from build123d import *

# Parameters (mm, degrees)
F1_DEPTH = 254
F2_T     = -2.54
F4_DEPTH = 25.4


with BuildPart() as f1:
    # F0 (on Right) → F1 (new body)
    with BuildSketch(Plane.YZ):
        with BuildLine():
            ThreePointArc((25.4, 19.05), (23.540128, 23.540128), (19.05, 25.4))
            Line((19.05, 25.4), (-19.05, 25.4))
            ThreePointArc((-19.05, 25.4), (-23.540128, 23.540128), (-25.4, 19.05))
            Line((-25.4, 19.05), (-25.4, -19.05))
            ThreePointArc((-25.4, -19.05), (-23.540128, -23.540128), (-19.05, -25.4))
            Line((-19.05, -25.4), (19.05, -25.4))
            ThreePointArc((19.05, -25.4), (23.540128, -23.540128), (25.4, -19.05))
            Line((25.4, -19.05), (25.4, 19.05))
        make_face()
    extrude(amount=F1_DEPTH)

    # F2
    f2_openings = [f1.faces().sort_by_distance(p)[0] for p in [
        (254, 0, 0),
        (0, 0, 0),
    ]]
    offset(amount=F2_T, openings=f2_openings)

    # F3 (on Front) → F4 (cut, symmetric)
    with BuildSketch(Plane.XZ):
        Polygon((254, 25.4), (190.5, 25.4), (241.3, -25.4), (254, -25.4), align=None)
    extrude(amount=F4_DEPTH, both=True, mode=Mode.SUBTRACT)


solid = f1.part
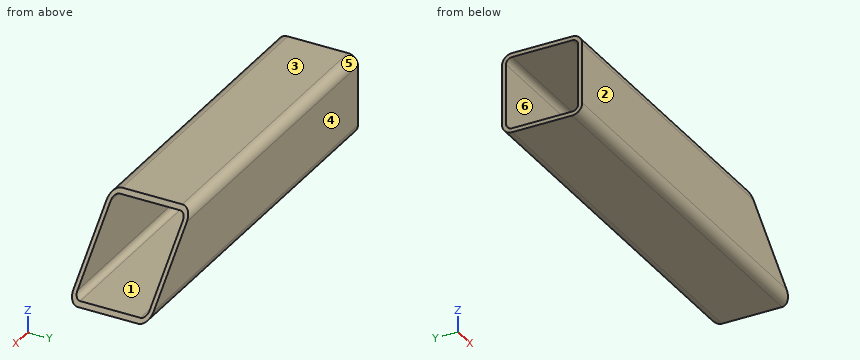
Can you work these out from the model? Positions are in its coordinate system, mm. Face numbers are marked on the shaded views. A direction names the side the tool comes from. Round coordinates to 2 decimals unless told otherwise and drop trailing zeros. Loops run counter-clockwise (first coordinate to the right, second up) from the corner with the lowest first, then second, coordinate; pieces in that order, holes last. Notation, with made-up numbers: (-30.75, 46) - (-13.75, 46) arc R23 cw to (-13.75, 70) - close; hole circle Ø2 at (-39.75, -25). An arc over 180 degrees is marked (long way). Answer in a Markdown table with one row per item. Add a question column.
Q1. I want a section at B-B on y = 16. List the corners of the cut face in (x, z) for me.
Q2. Which directions (+Z, -Z, +X, -X, +Y, -Y) give clear straight access to the entire face, cutting with the end or side of a thin tool? Please do the marked faces 5 and 6.
Q3. I need wall thicknesses on L1, parallel to Y at x = 57.5, z = 10.5; L2, parallel to Z at x = 138, y = -21. Which ranges of each line are inside material? Lowest first, please.
Q4. We'd pull the mould along Y, two halves only. Please class the marked faces 1, 2, 3 and 4: pulls with the +Y half, pulls with the -Y half, needs draft (parallel to the pull), parting line crosses it, or undercut.
Q5. I want a section at A-A on z = 4. List the corners of the cut face in (x, y) for me, and give its area (3 significant figures).
Q6. I want a section at C-C on x = 21. List the corners of the cut face in (y, z) for me, and give its area (3 significant figures).
A:
| question | item | result |
|---|---|---|
| 1 | outline | (0, -25.4) - (241.3, -25.4) - (238.76, -22.86) - (0, -22.86) - close; (0, 22.86) - (193.04, 22.86) - (190.5, 25.4) - (0, 25.4) - close |
| 2 | face 5 | +Z, +X, -X, +Y |
| 2 | face 6 | +X, -X |
| 3 | L1 | -25.4 to -22.86, 22.86 to 25.4 |
| 3 | L2 | -25.09 to -22.32, 22.32 to 25.09 |
| 4 | face 1 | undercut |
| 4 | face 2 | pulls with the -Y half |
| 4 | face 3 | needs draft |
| 4 | face 4 | pulls with the +Y half |
| 5 | outline | (0, -25.4) - (211.9, -25.4) - (211.9, -22.86) - (0, -22.86) - close; (0, 22.86) - (211.9, 22.86) - (211.9, 25.4) - (0, 25.4) - close |
| 5 | area | 1,080 mm^2 |
| 6 | outline | (-25.4, -19.05) arc R6.35 ccw to (-19.05, -25.4) - (19.05, -25.4) arc R6.35 ccw to (25.4, -19.05) - (25.4, 19.05) arc R6.35 ccw to (19.05, 25.4) - (-19.05, 25.4) arc R6.35 ccw to (-25.4, 19.05) - close; hole (-22.86, -19.05) arc R3.81 ccw to (-19.05, -22.86) - (19.05, -22.86) arc R3.81 ccw to (22.86, -19.05) - (22.86, 19.05) arc R3.81 ccw to (19.05, 22.86) - (-19.05, 22.86) arc R3.81 ccw to (-22.86, 19.05) - close |
| 6 | area | 468 mm^2 |
